Geometry: see drawing. Coordinates: mm, zero at the bounding-box minimum. Coordinates: 2 decimals unless noted, no trailing zeros. Loops run counter-clockwise (first coordinate to the right, second up) from the corner with the lowest first, then second, coordinate; pieces in that order, holes last. Notation, with made-up numbers: (46.25, 12.25) -> (76.25, 12.25) arc R31 cw to (76.25, 43.25) -> close; hole circle Ø7 at (33.5, 57.5). An arc over 180 degrees is marked (long way). Answer as a JSON object with one key per item and string values.
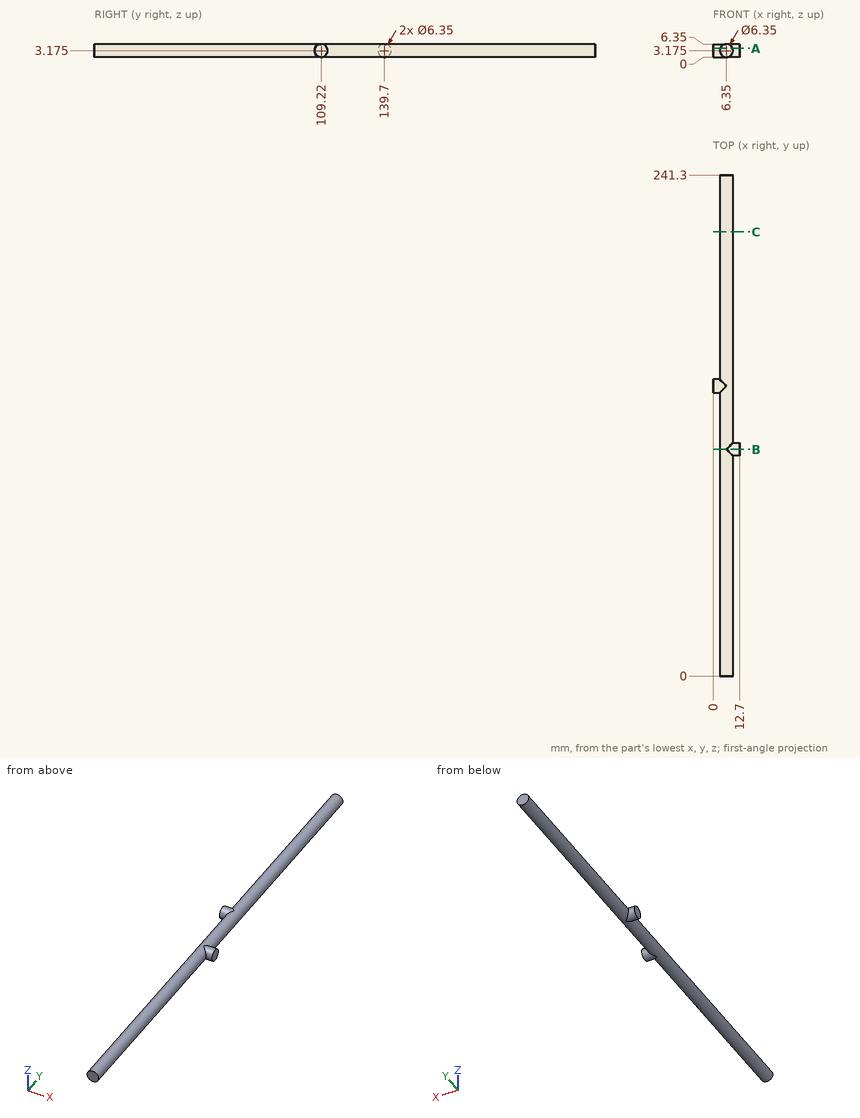
1. Section query C-C (y = 214). Return loops of the section in (x, z) (3 decimals).
Reply:
{"outline": "circle Ø6.35 at (6.35, 3.175)"}
2. Line query: line 1 along Z through (x, y) = (6.75, 58.5); line 2 along X through (y, z) = (150.5, 3.5); line 3 along Z through (x, y) = (3.5, 79). Output: solid intervals per line, ascending.
Reply:
{"line 1": "z = 0.03 to 6.32", "line 2": "x = 3.19 to 9.51", "line 3": "z = 1.78 to 4.57"}
3. Pin query (flat end, axial travel): P1, Ø2, axis at x = 5.5, y = 82.5, coming from the -Z side; P2, Ø3, axis at y = 191, z = 5, coming from the -X side; P3, Ø1, axis at x = 8, y = 98.5, coming from the +Z side; P4, Ø1, axis at y = 32, z = 3, coming from the +X side (3 decimals). Return the tip coordinate at first contact, or that it passes through.
Reply:
{"P1": "stops at z = 0", "P2": "stops at x = 3.19", "P3": "stops at z = 6.13", "P4": "stops at x = 9.525"}
4. Section query A-A (z = 4.25). Return loops of the section in (x, y), plus the area to 3 significant figures.
Reply:
{"outline": "(0, 136.71) -> (3.36, 136.71) -> (3.36, 0) -> (9.34, 0) -> (9.34, 106.23) -> (12.7, 106.23) -> (12.7, 112.21) -> (9.34, 112.21) -> (9.34, 241.3) -> (3.36, 241.3) -> (3.36, 142.69) -> (0, 142.69) -> close", "area": "1,480 mm2"}
5. Section query B-B (y = 109.22). Return loops of the section in (x, z) (3 decimals).
Reply:
{"outline": "(6.35, 0) -> (12.7, 0) -> (12.7, 6.35) -> (6.35, 6.35) arc R3.175 ccw to start"}
